Geometry check sheet. Reference: the model listing, model coordinates, mm. A direction names the side the tool comes from. Give positions to 0.01 mm unless a question says otherwise; leave off trailing zeros. Order: outer loops, then holes, each group sorted by start corner. A loop starts at its lowest first (then second) coordinate and runs counter-clockwise, first axis right, second up. Notation, with made-up numbers: M 71,-30 L 108,-30 A26 ccw 108,-8 Z; hole C -23.5,37 d4. An arc over 180 degrees is marked long. Answer as CSV lines item,"result". Start each with the question number.
Q1. Mould release check, pull along X, two halves, no side actions. Record for faces 3 (the flat face through (69.1, -117, -261.9)), 4 (the flat face through (111.558, -62.612, -198.184)), 5 (the conical face through (79.763, 7.5, -332.973)): +X half, -X half, draft (parallel to the pull), parting line (faces both ways), or undercut.
Q2. Section check A-A, the plane y = -40.5. Record the boundary of the cut face in (x, z), then the cut area to 3 significant figures.
Q3. Thickness scan on line 1 (Y direction, x = 14.5, z = -248); line 2 (Y direction, x = 45.5, z = -303); line 3 (X direction, y = -64.5, z = -280). Record the ranges inside material, lowest first.
Q4. Set-up check for faces 1 (the cylindrical face through (79.224, -53.625, -320.715)), 2 (the flat face through (112, 0, -325)): record each of +Z, -Z, +X, -X, +Y, -Y from which the full face is reachable in a straight line by a thin tool's end or side.
Q5. Go/stop test with flat-tipped pins: pin 1 (8 mm diameter, centred on y = -107, z = -228, fed in from +X); pin 2 (10 mm diameter, centred on x = 43, y = -24, fed in from -Z); pin 3 (6 mm diameter, centred on x = 135, y = -105, fed in from +Z). Record where each tip stops, or that it passes through.
```python
from build123d import *

# Parameters (mm, degrees)
SKETCH1_R           = 30
BOSS_EXTRUDE1_DEPTH = 127
BOSS_EXTRUDE2_START = 8
SKETCH3_R           = 45
SKETCH3_R_2         = 30
BOSS_EXTRUDE2_DEPTH = 8
CHAMFER1_SIZE2      = 8
CHAMFER1_SIZE       = 2.911761874
CUT_EXTRUDE1_START  = -10
SKETCH4_R           = 46
SKETCH4_R_2         = 30
CUT_EXTRUDE1_DEPTH  = 10
CHAMFER2_SIZE2      = 10
CHAMFER2_SIZE       = 3.639702343


# Some blends are built 0.0001 mm under size
with BuildPart() as part:
    # Sketch1 → Boss-Extrude1 (new body)
    with BuildSketch(Plane(origin=(0, 0, 0), x_dir=(1, 0, 0), z_dir=(0, 1, 0))):
        with BuildLine():
            Line((112.5, 194.855715851), (188.5, 326.491577227))
            ThreePointArc((188.5, 326.491577227), (97.574780004, 364.154036511), (0, 377))
            Line((0, 377), (0, 225))
            ThreePointArc((0, 225), (58.234285148, 217.333310915), (112.5, 194.855715851))
        make_face()
        with Locations(Location((77.904532576, 290.743673713, 0), (0, 0, 270))):
            Circle(SKETCH1_R, mode=Mode.SUBTRACT)
    extrude(amount=-BOSS_EXTRUDE1_DEPTH)

    # Sketch3 → Boss-Extrude2 (add)
    with BuildSketch(Plane(origin=(0, 0, 0), x_dir=(1, 0, 0), z_dir=(0, 1, 0)).offset(BOSS_EXTRUDE2_START)):
        with Locations(Location((77.904532576, 290.743673713, 0), (0, 0, 270))):
            Circle(SKETCH3_R)
        with Locations(Location((77.904532576, 290.743673713, 0), (0, 0, 270))):
            Circle(SKETCH3_R_2, mode=Mode.SUBTRACT)
    extrude(amount=-BOSS_EXTRUDE2_DEPTH)

    # Chamfer1
    chamfer1_edges = [part.edges().sort_by_distance(p)[0] for p in [
        (77.904532576, 8, -335.743673713),
    ]]
    chamfer1_side = [part.faces().sort_by_distance(p)[0] for p in [
        (77.904532576, 8, -335.685438476),
    ]]
    chamfer(chamfer1_edges, length=CHAMFER1_SIZE - 0.0001, length2=CHAMFER1_SIZE2 - 0.0001, reference=chamfer1_side[0])  # a hair under: the kernel refuses the full size

    # Sketch4 → Cut-Extrude1 (cut)
    with BuildSketch(Plane.XZ.offset(127).offset(CUT_EXTRUDE1_START)):
        with Locations(Location((77.904532576, -290.743673713, 0), (0, 0, 270))):
            Circle(SKETCH4_R)
        with Locations(Location((77.904532576, -290.743673713, 0), (0, 0, 90))):
            Circle(SKETCH4_R_2, mode=Mode.SUBTRACT)
    extrude(amount=CUT_EXTRUDE1_DEPTH, mode=Mode.SUBTRACT)

    # Chamfer2
    chamfer2_edges = [part.edges().sort_by_distance(p)[0] for p in [
        (77.904532576, -117, -244.743673713),
    ]]
    chamfer2_side = [part.faces().sort_by_distance(p)[0] for p in [
        (77.904532576, -117, -244.81646776),
    ]]
    chamfer(chamfer2_edges, length=CHAMFER2_SIZE - 0.0001, length2=CHAMFER2_SIZE2 - 0.0001, reference=chamfer2_side[0])  # a hair under: the kernel refuses the full size

    # Chamfer3
    # the kernel refuses this chamfer: 5 mm, written as the material it takes off along each edge
    with BuildSketch(Plane(origin=(0, -127, 0), x_dir=(0.5292424705918727, 0, -0.8484706284379036), z_dir=(0.8484706284379036, 0, 0.5292424705918727))) as chamfer3_piece_1:
        with BuildLine():
            Line((371.858578644, -0.141421356), (377.141421356, 5.141421356))
            Line((377.141421356, 5.141421356), (377.241421356, 5.141421356))
            ThreePointArc((377.241421356, 5.141421356), (377.1, 2.570710678), (377.1, 0))
            Line((377.1, 0), (377, -0.1))
            ThreePointArc((377, -0.1), (374.429289322, -0.1), (371.858578644, -0.241421356))
            Line((371.858578644, -0.241421356), (371.858578644, -0.141421356))
        make_face()
    revolve(axis=Axis((0, -127, 0), (0, 1, 0)), revolution_arc=33.908571791, mode=Mode.SUBTRACT)
    with BuildSketch(Plane(origin=(0, -127, 0), x_dir=(-0.05711995451760951, 0, -0.9983673225801746), z_dir=(-0.9983673225801746, 0, 0.05711995451760951))) as chamfer3_piece_2:
        with BuildLine():
            Line((230.141421356, 0.141421356), (224.858578644, -5.141421356))
            Line((224.858578644, -5.141421356), (224.758578644, -5.141421356))
            ThreePointArc((224.758578644, -5.141421356), (224.9, -2.570710678), (224.9, 0))
            Line((224.9, 0), (225, 0.1))
            ThreePointArc((225, 0.1), (227.570710678, 0.1), (230.141421356, 0.241421356))
            Line((230.141421356, 0.241421356), (230.141421356, 0.141421356))
        make_face()
    revolve(axis=Axis((0, -127, 0), (0, -1, 0)), revolution_arc=36.549029178, mode=Mode.SUBTRACT)
    with BuildSketch(Plane(origin=(0, 0, 0), x_dir=(0.5292424705918727, 0, -0.8484706284379036), z_dir=(0.8484706284379036, 0, 0.5292424705918727))) as chamfer3_piece_3:
        with BuildLine():
            Line((377.141421356, -5.141421356), (371.858578644, 0.141421356))
            Line((371.858578644, 0.141421356), (371.858578644, 0.241421356))
            ThreePointArc((371.858578644, 0.241421356), (374.429289322, 0.1), (377, 0.1))
            Line((377, 0.1), (377.1, 0))
            ThreePointArc((377.1, 0), (377.1, -2.570710678), (377.241421356, -5.141421356))
            Line((377.241421356, -5.141421356), (377.141421356, -5.141421356))
        make_face()
    revolve(axis=Axis((0, 0, 0), (0, 1, 0)), revolution_arc=33.908571791, mode=Mode.SUBTRACT)
    with BuildSketch(Plane(origin=(0, 0, 0), x_dir=(-0.05711995451760943, 0, -0.9983673225801746), z_dir=(-0.9983673225801746, 0, 0.05711995451760943))) as chamfer3_piece_4:
        with BuildLine():
            Line((224.858578644, 5.141421356), (230.141421356, -0.141421356))
            Line((230.141421356, -0.141421356), (230.141421356, -0.241421356))
            ThreePointArc((230.141421356, -0.241421356), (227.570710678, -0.1), (225, -0.1))
            Line((225, -0.1), (224.9, 0))
            ThreePointArc((224.9, 0), (224.9, 2.570710678), (224.758578644, 5.141421356))
            Line((224.758578644, 5.141421356), (224.858578644, 5.141421356))
        make_face()
    revolve(axis=Axis((0, 0, 0), (0, -1, 0)), revolution_arc=36.549029178, mode=Mode.SUBTRACT)
    with BuildSketch(Plane(origin=(0, 12.726295315, -225), x_dir=(-0.027477698296736765, 0, -0.9996224167636066), z_dir=(0, -1, 0))) as chamfer3_piece_5:
        with BuildLine():
            Line((5.090518126, 0), (-0.33429411, 5.023891374))
            Line((-0.33429411, 5.023891374), (-0.434172994, 5.018971161))
            ThreePointArc((-0.434172994, 5.018971161), (-0.183141977, 2.511326919), (-0.099962242, -0.00274777))
            Line((-0.099962242, -0.00274777), (0.00274777, -0.099962242))
            ThreePointArc((0.00274777, -0.099962242), (2.546085101, -0.030050788), (5.093265896, -0.099962242))
            Line((5.093265896, -0.099962242), (5.090518126, 0))
        make_face()
    extrude(amount=152.452590629, mode=Mode.SUBTRACT)
    with BuildSketch(Plane(origin=(0, 13.026648977, -377), x_dir=(-0.0275053668618043, 0, 0.9996216558247413), z_dir=(0, -1, 0))) as chamfer3_piece_6:
        with BuildLine():
            Line((5.176029718, 0), (-0.249663351, -5.204674974))
            Line((-0.249663351, -5.204674974), (-0.349653457, -5.203268263))
            ThreePointArc((-0.349653457, -5.203268263), (-0.162620276, -2.601558906), (-0.099962166, 0.002750537))
            Line((-0.099962166, 0.002750537), (0.002750537, 0.099962166))
            ThreePointArc((0.002750537, 0.099962166), (2.588807445, 0.0288048), (5.178780254, 0.099962166))
            Line((5.178780254, 0.099962166), (5.176029718, 0))
        make_face()
    extrude(amount=153.053297954, mode=Mode.SUBTRACT)
    with BuildSketch(Plane(origin=(188.5, 13.026648977, -326.491577227), x_dir=(-0.8556337629027079, 0, -0.5175817459889334), z_dir=(0, -1, 0))) as chamfer3_piece_7:
        with BuildLine():
            Line((5.210659591, 0), (-0.248004097, -5.170084874))
            Line((-0.248004097, -5.170084874), (-0.347983242, -5.168042668))
            ThreePointArc((-0.347983242, -5.168042668), (-0.152811741, -2.584453961), (-0.099979145, 0.002042206))
            Line((-0.099979145, 0.002042206), (0.002042206, 0.099979145))
            ThreePointArc((0.002042206, 0.099979145), (2.60636271, 0.037782504), (5.214045418, 0.099942664))
            Line((5.214045418, 0.099942664), (5.210659591, 0))
        make_face()
    extrude(amount=153.053297954, mode=Mode.SUBTRACT)
    with BuildSketch(Plane(origin=(112.5, 12.726295315, -194.855715851), x_dir=(-0.8848441204167522, 0, -0.46588719939906503), z_dir=(0, -1, 0))) as chamfer3_piece_8:
        with BuildLine():
            Line((5.0350012, 0), (-0.337980103, 5.0792858))
            Line((-0.337980103, 5.0792858), (-0.437904212, 5.075390609))
            ThreePointArc((-0.437904212, 5.075390609), (-0.199029377, 2.538471922), (-0.099924109, -0.003895191))
            Line((-0.099924109, -0.003895191), (0.003895191, -0.099924109))
            ThreePointArc((0.003895191, -0.099924109), (2.517945165, -0.016000711), (5.036723207, -0.099985172))
            Line((5.036723207, -0.099985172), (5.0350012, 0))
        make_face()
    extrude(amount=152.452590629, mode=Mode.SUBTRACT)


solid = part.part
```
Answer block:
1,face 3,"undercut"
1,face 4,"+X half"
1,face 5,"parting line"
2,outline,"M 0,-371.97 L 5.07,-376.97 A377 ccw 184.09,-329 L 185.98,-322.13 L 114.97,-199.14 L 108.24,-197.26 A225 cw 4.89,-224.95 L 0,-229.95 Z; hole C 77.9,-290.74 d60"
2,area,"21,100 mm2"
3,line 1,"y = -127 to 0"
3,line 2,"y = -117 to 8"
3,line 3,"x = 0 to 49.89, 105.91 to 161.66"
4,face 1,"+Y, -Y"
4,face 2,"+Y"
5,pin 1,"stops at x = 133.95"
5,pin 2,"stops at z = -375.08"
5,pin 3,"stops at z = -228.63"
